from build123d import *

# Parameters (mm, degrees)
F0_W     = 198.4809562564
F0_H     = 112.2947335243
F1_DEPTH = 39.878
F2_R     = 20.7776097732
F3_DEPTH = 15.748
F4_W     = 198.4809562564
F4_H     = 112.2947335243
F4_R     = 20.7776097732
F5_DEPTH = 21.336
F6_ANGLE = 180
F7_T     = -2.54


with BuildPart() as f1:
    # F0 (on Top) → F1 (new body)
    with BuildSketch(Plane.XY):
        with Locations((0.2176724374, -0.7018409669)):
            Rectangle(F0_W, F0_H)
    extrude(amount=F1_DEPTH)

    # F2 (on face) → F3 (join)
    with BuildSketch(Plane(origin=(0, 0, 0), x_dir=(1, 0, 0), z_dir=(0, 0, -1))):
        with Locations((-61.0377900302, 27.6237465441)):
            Circle(F2_R)
        with Locations((-60.1607970893, -27.2515378892)):
            Circle(F2_R)
        with Locations((0, -25.1830536872)):
            Circle(F2_R)
        with Locations((0, 27.1037101871)):
            Circle(F2_R)
        with Locations((60.9036274254, -24.7248988599)):
            Circle(F2_R)
        with Locations((59.5011785626, 26.3048261404)):
            Circle(F2_R)
    extrude(amount=F3_DEPTH)

    # F4 (on face) → F5 (join)
    with BuildSketch(Plane.XY.offset(39.878)):
        with Locations((0.2176724374, -0.7018409669)):
            Rectangle(F4_W, F4_H)
        with Locations((-59.3232288957, -28.0555449426)):
            Circle(F4_R, mode=Mode.SUBTRACT)
        with Locations((0, -27.5396611542)):
            Circle(F4_R, mode=Mode.SUBTRACT)
        with Locations((60.3502318263, -27.691854164)):
            Circle(F4_R, mode=Mode.SUBTRACT)
        with Locations((-59.7541630268, 26.5966858715)):
            Circle(F4_R, mode=Mode.SUBTRACT)
        with Locations((0, 28.0189700425)):
            Circle(F4_R, mode=Mode.SUBTRACT)
        with Locations((61.206471175, 27.1779913455)):
            Circle(F4_R, mode=Mode.SUBTRACT)
    extrude(amount=F5_DEPTH)


with BuildPart() as f1_1:
    # F6: moved
    add(f1.part.rotate(Axis((0.2176724374, -56.8492077291, 61.214), (1, 0, 0)), F6_ANGLE))

    # F7
    f7_openings = [f1_1.faces().sort_by_distance(p)[0] for p in [
        (-60.160797, -140.949953, 138.176),
        (-61.03779, -86.074669, 138.176),
        (0, -86.594705, 138.176),
        (0, -138.881469, 138.176),
        (60.903627, -138.423314, 138.176),
        (59.501179, -87.393589, 138.176),
    ]]
    offset(amount=F7_T, openings=f7_openings, kind=Kind.INTERSECTION)


solid = f1_1.part
Part model, mm, in its own coordinate system. A direction names the side the tool comes from. Coordinates: 2 decimals unless noted, no trailing zeros. Order: outer loops, then holes, each group sorted by start corner. A loop starts at its lowest first (then second) coordinate and runs counter-clockwise, first axis right, second up. Notation, with made-up numbers: M -0.75,83.25 L 47.25,83.25 A26 ccw 47.25,110.25 Z; hole C -12.75,-15.5 d10. An arc over 180 degrees is marked long. Use a Markdown table: item, result.
(1) Cut at A-A on z = 70. State how many separate pieces and enclosed holes the cut face has, then the cut area to 3 significant figures.
A:
| item | result |
|---|---|
| separate pieces | 7 |
| enclosed holes | 7 |
| area | 3,660 mm^2 |
(2) Probe L1, parallel to Y at x = 0, z = 66.5 (3 decimals); L2, parallel to Z at x = -84.5, y = -124; L3, parallel to X at y = -79.5, z = 92. List the from-to ranges inside material, lowest first.
A:
| item | result |
|---|---|
| L1 | y = -169.144 to -166.604, -165.035 to -162.495, -120.94 to -118.4, -109.476 to -106.936, -65.381 to -62.841, -59.389 to -56.849 |
| L2 | z = 61.21 to 63.75, 119.89 to 122.43 |
| L3 | x = -99.02 to -96.48, 96.92 to 99.46 |
(3) Pull direction Z, two halves, no side cores. Call faces 4 (the cylindrical face through (82.59, -93.01, 74.57)), 5 (the flat face through (61, -141, 85.09)), 6 (the cylindrical face through (11.17, -159.237, 72.031)): released by +Z, released by -Z, zero draft, split by the parting line, or undercut.
A:
| item | result |
|---|---|
| face 4 | undercut |
| face 5 | undercut |
| face 6 | zero draft |
(4) Tool access for faces 1 (the cylindrical face through (-4.5, -106.88, 130.19)), 2 (the flat face through (60, -86, 85.09)), 3 (the cylindrical face through (79.543, -78.049, 72.031)): list every direction of +Z, -Z, +X, -X, +Y, -Y with a clear straight run to the whole face (end or side of a thin tool).
A:
| item | result |
|---|---|
| face 1 | +Z |
| face 2 | none |
| face 3 | -Z |
(5) Cut at B-B on z = 111.5. Write the cut outline in (x, y).
A:
| item | result |
|---|---|
| outline | M -99.02,-169.14 L 99.46,-169.14 L 99.46,-56.85 L -99.02,-56.85 Z; hole M -96.48,-166.6 L 96.92,-166.6 L 96.92,-59.39 L -96.48,-59.39 Z |
(6) Flat gauge pins, fed straight in: pin 1 (4 mm diameter, centred on x = 30, y = -140.5, fed in from +Z); pin 2 (3 mm diameter, centred on y = -138, z = 127.5, fed in from +X); pin 3 (14 mm diameter, centred on x = 56, y = -148.5, fed in from +Z). Where does each tip first touch, or does it go through?
A:
| item | result |
|---|---|
| pin 1 | stops at z = 122.43 |
| pin 2 | stops at x = 81.68 |
| pin 3 | stops at z = 85.09 |
